Check sheet for the modelled part. Datum: model origin and axes. Units: mm. Face numbers are marked on the shaded views. Give positions to 0.01 mm unless a question says otherwise; leave off trailing zeros. Order: outer loops, then holes, each group sorted by start corner. A loop starts at its lowest first (then second) coordinate and runs counter-clockwise, first axis right, second up. Notation, with made-up numbers: (79, 33) -> (137, 33) arc R8 cw to (137, 39) -> close; hole circle Ø10 at (85.5, 61.25). An arc over 180 degrees is marked (long way). Write each question's results on one line, items separated by ' | '.
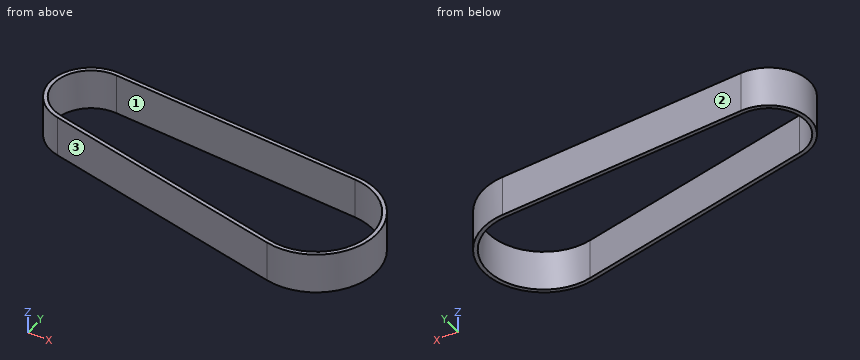
from build123d import *

# Parameters (mm, degrees)
CROQUIS3_W = 10
CROQUIS3_H = 1


with BuildPart() as part:
    # Barrer1: sweep along a path in Croquis2
    with BuildLine(Plane.XY) as barrer1_path:
        Line((0.659407884, 9.106156228), (62.491462424, 4.628685909))
        ThreePointArc((62.491462424, 4.628685909), (75.23778781, -11.306375083), (58.370917042, -22.79130652))
        Line((58.370917042, -22.79130652), (-2.046135399, -8.897765446))
        ThreePointArc((-2.046135399, -8.897765446), (-9.028624048, 1.356778461), (0.659407884, 9.106156228))
    # Croquis3 → Barrer1 (sweep)
    with BuildSketch(Plane(origin=(0.659407884, 0, 0), x_dir=(0, 0, -1), z_dir=(1, 0, 0))):
        with Locations((0, 9.606156228)):
            Rectangle(CROQUIS3_W, CROQUIS3_H)
    sweep(path=barrer1_path.line)


solid = part.part
1. Gauge pin test, flat ends, axial feed: pin 1 Ø4 at (y, z) = (6.5, 2.5) entering from +X; pin 2 Ø2 at (y, z) = (1.5, 3) entering from -X; pin 3 Ø6 at (y, z) = (-20, -0.5) entering from +X. Record the tip position at first contact, or that the pin passes through.
Verdict:
pin 1: stops at x = 67.26 | pin 2: stops at x = -10.12 | pin 3: stops at x = 74.21
2. Section check A-A on z = -4. Record the cut outline in (x, y) (3 decimals), then the cut area to 3 significant figures.
Verdict:
outline: (-2.199, -9.886) -> (58.218, -23.78) arc R14.903 ccw (long way) to (62.491, 5.629) -> (0.659, 10.106) arc R10.128 ccw to start; hole (-2.046, -8.898) -> (58.371, -22.791) arc R13.905 ccw (long way) to (62.491, 4.629) -> (0.659, 9.106) arc R9.13 ccw to start | area: 200 mm^2
3. Mould release check, pull along X, two halves, no side actions. Record for the marked faces 1, 2 and 3: +X half, -X half, draft (parallel to the pull), parting line (faces both ways), or undercut.
Verdict:
face 1: undercut | face 2: +X half | face 3: -X half
4. Section check C-C on y = -12. Record the cut outline in (x, z).
Verdict:
outline: (6.99, -5) -> (11.44, -5) -> (11.44, 5) -> (6.99, 5) -> close; (75.12, -5) -> (76.13, -5) -> (76.13, 5) -> (75.12, 5) -> close
5. Material ranges on probe 1 along X at (y, z) = (-1, 3.75); probe 2 along X at (y, z) = (2, 3); probe 3 along Y at (x, z) = (51.5, 1), recorded low to high. Write a range as from..to.
Verdict:
probe 1: x = -10.08..-9.08, 72.69..73.9 | probe 2: x = -9.93..-8.91, 69.67..71.27 | probe 3: y = -22.23..-21.21, 5.42..6.42
6. Section check B-B on y = -2. Record the cut outline in (x, z), then the cut area to 3 significant figures.
Verdict:
outline: (-9.93, -5) -> (-8.91, -5) -> (-8.91, 5) -> (-9.93, 5) -> close; (73.36, -5) -> (74.51, -5) -> (74.51, 5) -> (73.36, 5) -> close | area: 21.7 mm^2
